from build123d import *

# Parameters (mm, degrees)
SKETCH1_R           = 4
BOSS_EXTRUDE1_DEPTH = 2.5


with BuildPart() as part:
    # Sketch1 → Boss-Extrude1 (new, symmetric)
    with BuildSketch(Plane.YZ):
        with BuildLine():
            Line((-29.297384522, 51.898953809), (-40.5, 0))
            Line((-40.5, 0), (-25.5, 0))
            Line((-25.5, 0), (-25.5, -5))
            Line((-25.5, -5), (-15.5, -5))
            Line((-15.5, -5), (-15.5, 0))
            Line((-15.5, 0), (15.5, 0))
            Line((15.5, 0), (15.5, -5))
            Line((15.5, -5), (25.5, -5))
            Line((25.5, -5), (25.5, 0))
            Line((25.5, 0), (40.5, 0))
            Line((40.5, 0), (28.085365409, 61.773282105))
            ThreePointArc((28.085365409, 61.773282105), (24.06562356, 67.610728604), (17.066668753, 68.728197959))
            Line((17.066668753, 68.728197959), (-22.695121951, 58.728197959))
            ThreePointArc((-22.695121951, 58.728197959), (-26.970582938, 56.255522076), (-29.297384522, 51.898953809))
        make_face()
        with Locations(Location((-20.5, 50, 0), (0, 0, 270))):
            Circle(SKETCH1_R, mode=Mode.SUBTRACT)
        with Locations(Location((19.261790704, 60, 0), (0, 0, 270))):
            Circle(SKETCH1_R, mode=Mode.SUBTRACT)
    extrude(amount=BOSS_EXTRUDE1_DEPTH, both=True)


solid = part.part
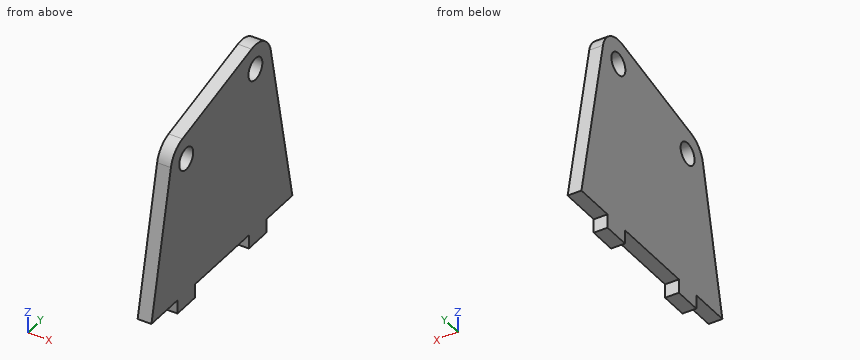
The model under review builds one solid part; all positions refer to its coordinate system, in mm. Round coordinates to 2 decimals unless told otherwise and drop trailing zeros. Loops run counter-clockwise (first coordinate to the right, second up) from the corner with the lowest first, then second, coordinate; pieces in that order, holes last. Notation, with made-up numbers: M 62.25,73 L 102.25,73 A16 cw 102.25,87 Z; hole C -5.5,10 d9. An arc over 180 degrees is marked long. Answer as a JSON object with one key per item and string values.
Item 1: We need section A-A, the plane z = 60. State the section outline as (x, y) points.
Check sheet entries:
{"outline": "M -2.5,-17.64 L 2.5,-17.64 L 2.5,15.26 L -2.5,15.26 Z; M -2.5,23.26 L 2.5,23.26 L 2.5,28.44 L -2.5,28.44 Z"}
Item 2: Clearance check with flat-ended pins moving along their axes: P1, Ø1, axis at x = 2, y = -21.5, coming from the +Z side; P2, Ø6.5, axis at y = -20.5, z = 50, coming from the -X side; P3, Ø1.5, axis at x = -1, z = 61.5, coming from the +Y side; P4, Ø1, axis at x = 2, y = -3.5, coming from the -Z side. State where each tip first meets the part, or that it passes through.
Check sheet entries:
{"P1": "z = 59.15", "P2": "through", "P3": "y = 28.29", "P4": "z = 0"}
Item 3: For line 1 along Z through (x, y) = (0.65, 1.5); line 2 along Z through (x, y) = (-0.2, 18); line 3 along Z through (x, y) = (0.7, 15), list the stretches that pass through material, from the lowest coordinate up.
Check sheet entries:
{"line 1": "0 to 64.81", "line 2": "-5 to 56.2, 63.8 to 68.91", "line 3": "0 to 68.21"}
Item 4: We need section C-C, the plane y = -20.5. State the section outline as (x, z) points.
Check sheet entries:
{"outline": "M -2.5,-5 L 2.5,-5 L 2.5,46 L -2.5,46 Z; M -2.5,54 L 2.5,54 L 2.5,59.28 L -2.5,59.28 Z"}
Item 5: We need section B-B, the plane x = 0.75. State the section outline as (y, z) points, and give its area (3 significant figures).
Check sheet entries:
{"outline": "M -40.5,0 L -25.5,0 L -25.5,-5 L -15.5,-5 L -15.5,0 L 15.5,0 L 15.5,-5 L 25.5,-5 L 25.5,0 L 40.5,0 L 28.09,61.77 A9 ccw 17.07,68.73 L -22.7,58.73 A9 ccw -29.3,51.9 Z; hole C -20.5,50 d8; hole C 19.26,60 d8", "area": "4,330 mm2"}
Item 6: We need section D-D, the plane z = 25.5. State the section outline as (x, y) points.
Check sheet entries:
{"outline": "M -2.5,-35 L 2.5,-35 L 2.5,35.38 L -2.5,35.38 Z"}
